```python
from build123d import *

# Parameters (mm, degrees)
SKETCH1_R             = 141.5
SKETCH1_R_2           = 131.5
BOSS_EXTRUDE2_DEPTH   = 5
SKETCH1_R_3           = 152.5
SKETCH1_R_4           = 142.5
BOSS_EXTRUDE2_2_DEPTH = 5
SKETCH1_4_R           = 142.5
SKETCH1_4_R_2         = 141.5
BOSS_EXTRUDE3_DEPTH   = 4
SKETCH2_R             = 1.5
CUT_EXTRUDE1_DEPTH    = 4


with BuildPart() as part:
    # Sketch1 → Boss-Extrude2 (new, symmetric)
    with BuildSketch(Plane(origin=(0, 0, 0), x_dir=(0, 0, -1), z_dir=(1, 0, 0))):
        Circle(SKETCH1_R)
        Circle(SKETCH1_R_2, mode=Mode.SUBTRACT)
    extrude(amount=BOSS_EXTRUDE2_DEPTH, both=True)



with BuildPart() as body_2:
    # Sketch1 → Boss-Extrude2 2 (new, symmetric)
    with BuildSketch(Plane(origin=(0, 0, 0), x_dir=(0, 0, -1), z_dir=(1, 0, 0))):
        Circle(SKETCH1_R_3)
        Circle(SKETCH1_R_4, mode=Mode.SUBTRACT)
    extrude(amount=BOSS_EXTRUDE2_2_DEPTH, both=True)


with BuildPart() as part_1:
    add(part.part)

    add(body_2.part)  # Boss-Extrude3 merges body 2
    # Sketch1_4 → Boss-Extrude3 (add, symmetric)
    with BuildSketch(Plane(origin=(0, 0, 0), x_dir=(0, 0, -1), z_dir=(1, 0, 0))):
        Circle(SKETCH1_4_R)
        Circle(SKETCH1_4_R_2, mode=Mode.SUBTRACT)
    extrude(amount=BOSS_EXTRUDE3_DEPTH, both=True)

    # Sketch2 → Cut-Extrude1 (cut)
    with BuildSketch(Plane(origin=(5, 0, 0), x_dir=(0, 0, -1), z_dir=(1, 0, 0))):
        with Locations((0, 136.5)):
            Circle(SKETCH2_R)
        with Locations((118.212467617, -68.25)):
            Circle(SKETCH2_R)
        with Locations((-118.212467617, -68.25)):
            Circle(SKETCH2_R)
    extrude(amount=-CUT_EXTRUDE1_DEPTH, mode=Mode.SUBTRACT)


solid = part_1.part
```
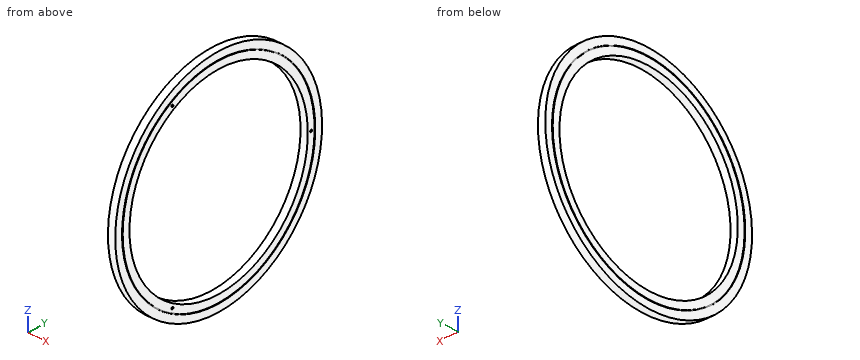
Check sheet for the modelled part. Datum: model origin and axes. Units: mm. Give positions to 0.01 mm unless a question says otherwise; leave off trailing zeros. Loops run counter-clockwise (first coordinate to the right, second up) from the corner with the lowest first, then second, coordinate; pieces in that order, holes last. Notation, with made-up numbers: M -24,-32.75 L 32,-32.75 A17 ccw 32,-1.75 Z; hole C 17,-25 d1. An arc over 180 degrees is marked long. Answer in a Markdown table with one row per item.
1) Thickness scan on line 1 (Y direction, x = -4.4, z = 0); line 2 (Z direction, x = 2.1, y = -68.25); line 3 (Y direction, x = -4.25, z = 99.5). Record the ranges inside material, lowest first.
Solutions:
| item | result |
|---|---|
| line 1 | y = -152.5 to -142.5, -141.5 to -131.5, 131.5 to 141.5, 142.5 to 152.5 |
| line 2 | z = -136.38 to -119.71, -116.71 to -112.4, 112.4 to 116.71, 119.71 to 136.38 |
| line 3 | y = -115.57 to -102.01, -100.61 to -85.98, 85.98 to 100.61, 102.01 to 115.57 |
2) Cross-section at C-C (x = 2.5). Enter the section's corners in (y, z).
Solutions:
| item | result |
|---|---|
| outline | C 0,0 d305; hole C 0,0 d263; hole C -68.25,-118.21 d3; hole C -68.25,118.21 d3; hole C 136.5,0 d3 |
3) Cross-section at A-A (y = -116.5). Enter the section's corners in (x, z).
Solutions:
| item | result |
|---|---|
| outline | M -5,-98.41 L 5,-98.41 L 5,-82.06 L 4,-82.06 L 4,-80.31 L 5,-80.31 L 5,-60.99 L -5,-60.99 L -5,-80.31 L -4,-80.31 L -4,-82.06 L -5,-82.06 Z; M -5,60.99 L 5,60.99 L 5,80.31 L 4,80.31 L 4,82.06 L 5,82.06 L 5,98.41 L -5,98.41 L -5,82.06 L -4,82.06 L -4,80.31 L -5,80.31 Z |
4) Depth check by flat-ended pin: pin 1 (4 mm diameter, centred on x = 2.5, z = 59.5, fed in from +Y); pin 2 (5 mm diameter, centred on x = 3, z = 45, fed in from +Y); pin 3 (2.5 mm diameter, centred on y = 136.5, z = 0, fed in from +X). Enter the tip coordinate at first touch or a pass-through.
Solutions:
| item | result |
|---|---|
| pin 1 | stops at y = 141.24 |
| pin 2 | stops at y = 146.46 |
| pin 3 | stops at x = 1 |
5) Cross-section at B-B (z = 66). Enter the section's corners in (x, y), plus the area to 3 significant figures.
Solutions:
| item | result |
|---|---|
| outline | M -5,-137.48 L 5,-137.48 L 5,-126.29 L 4,-126.29 L 4,-125.16 L 5,-125.16 L 5,-113.74 L -5,-113.74 L -5,-125.16 L -4,-125.16 L -4,-126.29 L -5,-126.29 Z; M -5,113.74 L 5,113.74 L 5,125.16 L 4,125.16 L 4,126.29 L 5,126.29 L 5,137.48 L -5,137.48 L -5,126.29 L -4,126.29 L -4,125.16 L -5,125.16 Z |
| area | 470 mm^2 |
